```python
from build123d import *

# Parameters (mm, degrees)
F1_DEPTH = 40
F3_W     = 10
F3_H     = 9.5
F4_DEPTH = 2
F5_DEPTH = 30
F6_W     = 1.5
F6_H     = 4
F7_DEPTH = 9.501
F8_SIZE  = 2.49999


# Not quite as in the source:
# - a fillet or chamfer is up to 0.001 mm smaller than in the source, because OpenCascade refuses the exact size


with BuildPart() as f1:
    # F0 (on Top) → F1 (new body)
    with BuildSketch(Plane.XY):
        with BuildLine():
            Line((-9.5, 0), (-8, 0))
            ThreePointArc((-8, 0), (0, 8), (8, 0))
            Line((8, 0), (9.5, 0))
            Line((9.5, 0), (9.5, 9.5))
            Line((9.5, 9.5), (-9.5, 9.5))
            Line((-9.5, 9.5), (-9.5, 0))
        make_face()
    extrude(amount=-F1_DEPTH)

    # F3 (on offset) → F4 (join)
    with BuildSketch(Plane.XY.offset(-10)):
        with Locations((-14.5, 4.75)):
            Rectangle(F3_W, F3_H)
        with Locations((14.5, 4.75)):
            Rectangle(F3_W, F3_H)
    extrude(amount=F4_DEPTH)

    # F5 (add): a face of the model
    f5_faces = [f1.faces().sort_by_distance(p)[0] for p in [
        (-8.75, 0.2124264579, 0),
    ]]
    extrude(f5_faces, amount=F5_DEPTH)

    # F6 (on face) → F7 (cut, through all)
    with BuildSketch(Plane.XZ):
        with Locations((-8.75, -3.5)):
            Rectangle(F6_W, F6_H)
        with Locations((-8.75, -35)):
            Rectangle(F6_W, F6_H)
        with Locations((8.75, -3.5)):
            Rectangle(F6_W, F6_H)
        with Locations((8.75, -35)):
            Rectangle(F6_W, F6_H)
        with Locations((-8.75, 25)):
            Rectangle(F6_W, F6_H)
        with Locations((8.75, 25)):
            Rectangle(F6_W, F6_H)
        with Locations((-8.75, 10.75)):
            Rectangle(F6_W, F6_H)
        with Locations((8.75, 10.75)):
            Rectangle(F6_W, F6_H)
    extrude(amount=-F7_DEPTH, mode=Mode.SUBTRACT)

    # F8 (size 2.5 in the source; OpenCascade refuses exactly that, so slightly less here)
    f8_edges = [f1.edges().sort_by_distance(p)[0] for p in [
        (-9.5, 4.75, -8),
        (9.5, 4.75, -8),
    ]]
    chamfer(f8_edges, length=F8_SIZE)


solid = f1.part
```
The listing builds one solid part. Answer for the finished solid, in the listing's coordinates (mm). A direction names the side the tool comes from. Round coordinates to 2 decimals unless told otherwise and drop trailing zeros. Order: outer loops, then holes, each group sorted by start corner. A loop starts at its lowest first (then second) coordinate and runs counter-clockwise, first axis right, second up. Notation, with made-up numbers: (-35.5, -39) -> (-23.5, -39) arc R17 ccw to (-23.5, -35) -> close; hole circle Ø4 at (23, 74.25). An arc over 180 degrees is marked (long way). Answer as CSV lines item,"result".
Q1. A cutting plane is placed at B-B on x = -14. Determine the outline of the cut face in (y, z).
Computed values:
outline,"(0, -10) -> (9.5, -10) -> (9.5, -8) -> (0, -8) -> close"
Q2. Given pin 1 (2 mm diameter, centred on y = 3.5, z = -35, fed in from -X); pin 2 (3 mm diameter, centred on y = 4.5, z = 10, fed in from -X); pin 3 (1.5 mm diameter, centred on y = 3, z = 18, fed in from +X), each flat-ended and moving along its own axis, determine where each tip first touches the part or whether it passes through.
Computed values:
pin 1,"stops at x = -8"
pin 2,"stops at x = -9.5"
pin 3,"stops at x = 9.5"
Q3. Consider line 1 (Z direction, x = 17.5, y = 4.5); line 2 (X direction, y = 1.75, z = 6); line 3 (X direction, y = 2, z = -14.5). Determine where each line is inside the solid, lowest interval first. Write a range as from..to.
Computed values:
line 1,"z = -10..-8"
line 2,"x = -9.5..-7.81, 7.81..9.5"
line 3,"x = -9.5..-7.75, 7.75..9.5"
Q4. Which of the six approach directions +Z, -Z, +X, -X, +Y, -Y give full straight-line access (tool end or side, diameter ignored) to faces 1 (the flat face through (9.5, 5, 4)), 2 (the flat face through (9.5, 5, -21)), 3 (the flat face through (9, 5, -1.5))?
Computed values:
face 1,"+Z, +X, +Y, -Y"
face 2,"-Z, +X, +Y, -Y"
face 3,"+X, +Y, -Y"
Q5. A cutting plane is placed at A-A on z = -13.5. Determine the outline of the cut face in (x, y), plus the area to 3 significant figures.
Computed values:
outline,"(-9.5, 0) -> (-8, 0) arc R8 cw to (8, 0) -> (9.5, 0) -> (9.5, 9.5) -> (-9.5, 9.5) -> close"
area,"80.0 mm^2"
Q6. A cutting plane is placed at C-C on x = 0. Determine the outline of the cut face in (y, z), plus the area to 3 significant figures.
Computed values:
outline,"(8, -40) -> (9.5, -40) -> (9.5, 30) -> (8, 30) -> close"
area,"105 mm^2"
